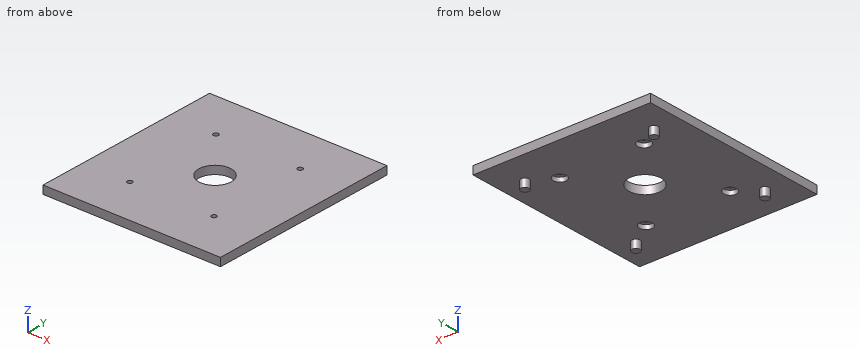
from build123d import *

# Parameters (mm, degrees)
F0_W           = 139.7
F0_H           = 152.4
F0_R           = 3.175
F0_R_2         = 1.984375
F0_R_3         = 12.7
F1_DEPTH       = 6.35
F2_R           = 3.175
F3_DEPTH       = 12.7
F5_D           = 3.9624
F5_CBORE_D     = 10.31875
F5_CBORE_DEPTH = 3.3734375


with BuildPart() as f1:
    # F0 (on Top) → F1 (new body)
    with BuildSketch(Plane.XY):
        Rectangle(F0_W, F0_H)
        with Locations((-50.8, -50.8)):
            Circle(F0_R, mode=Mode.SUBTRACT)
        with Locations((-25.4, -50.8)):
            Circle(F0_R, mode=Mode.SUBTRACT)
        with Locations((-33.1390625, -39.38984375)):
            Circle(F0_R_2, mode=Mode.SUBTRACT)
        with Locations((-50.8, -25.4)):
            Circle(F0_R, mode=Mode.SUBTRACT)
        with Locations((-25.4, -25.4)):
            Circle(F0_R, mode=Mode.SUBTRACT)
        with Locations((0, -50.8)):
            Circle(F0_R, mode=Mode.SUBTRACT)
        with Locations((25.4, -50.8)):
            Circle(F0_R, mode=Mode.SUBTRACT)
        with Locations((33.1390625, -39.38984375)):
            Circle(F0_R_2, mode=Mode.SUBTRACT)
        with Locations((50.8, -50.8)):
            Circle(F0_R, mode=Mode.SUBTRACT)
        with Locations((0, -25.4)):
            Circle(F0_R, mode=Mode.SUBTRACT)
        with Locations((25.4, -25.4)):
            Circle(F0_R, mode=Mode.SUBTRACT)
        with Locations((50.8, -25.4)):
            Circle(F0_R, mode=Mode.SUBTRACT)
        with Locations((-50.8, 0)):
            Circle(F0_R, mode=Mode.SUBTRACT)
        with Locations((-50.8, 25.4)):
            Circle(F0_R, mode=Mode.SUBTRACT)
        with Locations((-25.4, 0)):
            Circle(F0_R, mode=Mode.SUBTRACT)
        with Locations((-25.4, 25.4)):
            Circle(F0_R, mode=Mode.SUBTRACT)
        with Locations((-50.8, 50.8)):
            Circle(F0_R, mode=Mode.SUBTRACT)
        with Locations((-33.1390625, 39.38984375)):
            Circle(F0_R_2, mode=Mode.SUBTRACT)
        with Locations((-25.4, 50.8)):
            Circle(F0_R, mode=Mode.SUBTRACT)
        Circle(F0_R_3, mode=Mode.SUBTRACT)
        with Locations((25.4, 0)):
            Circle(F0_R, mode=Mode.SUBTRACT)
        with Locations((0, 25.4)):
            Circle(F0_R, mode=Mode.SUBTRACT)
        with Locations((25.4, 25.4)):
            Circle(F0_R, mode=Mode.SUBTRACT)
        with Locations((50.8, 0)):
            Circle(F0_R, mode=Mode.SUBTRACT)
        with Locations((50.8, 25.4)):
            Circle(F0_R, mode=Mode.SUBTRACT)
        with Locations((0, 50.8)):
            Circle(F0_R, mode=Mode.SUBTRACT)
        with Locations((33.1390625, 39.38984375)):
            Circle(F0_R_2, mode=Mode.SUBTRACT)
        with Locations((25.4, 50.8)):
            Circle(F0_R, mode=Mode.SUBTRACT)
        with Locations((50.8, 50.8)):
            Circle(F0_R, mode=Mode.SUBTRACT)
        with Locations((-25.4, 50.8)):
            Circle(F0_R)
        with Locations((0, 50.8)):
            Circle(F0_R)
        with Locations((25.4, 50.8)):
            Circle(F0_R)
        with Locations((50.8, 25.4)):
            Circle(F0_R)
        with Locations((50.8, 0)):
            Circle(F0_R)
        with Locations((50.8, -25.4)):
            Circle(F0_R)
        with Locations((25.4, -50.8)):
            Circle(F0_R)
        with Locations((0, -50.8)):
            Circle(F0_R)
        with Locations((-25.4, -50.8)):
            Circle(F0_R)
        with Locations((-50.8, -25.4)):
            Circle(F0_R)
        with Locations((-50.8, 0)):
            Circle(F0_R)
        with Locations((-50.8, 25.4)):
            Circle(F0_R)
        with Locations((-25.4, 25.4)):
            Circle(F0_R)
        with Locations((0, 25.4)):
            Circle(F0_R)
        with Locations((25.4, 25.4)):
            Circle(F0_R)
        with Locations((25.4, 0)):
            Circle(F0_R)
        with Locations((25.4, -25.4)):
            Circle(F0_R)
        with Locations((0, -25.4)):
            Circle(F0_R)
        with Locations((-25.4, 0)):
            Circle(F0_R)
        with Locations((-25.4, -25.4)):
            Circle(F0_R)
    extrude(amount=F1_DEPTH)

    # F2 (on face) → F3 (join)
    with BuildSketch(Plane.XY.offset(6.35)):
        with Locations((50.8, -50.8)):
            Circle(F2_R)
        with Locations((-50.8, -50.8)):
            Circle(F2_R)
        with Locations((-50.8, 50.8)):
            Circle(F2_R)
        with Locations((50.8, 50.8)):
            Circle(F2_R)
    extrude(amount=-F3_DEPTH)

    # F5 (through all)
    with Locations(Plane(origin=(0, 0, 0), x_dir=(1, 0, 0), z_dir=(0, 0, -1))):
        with Locations((-33.1390625, 39.38984375), (33.1390625, 39.38984375), (33.1390625, -39.38984375), (-33.1390625, -39.38984375)):
            CounterBoreHole(F5_D / 2, F5_CBORE_D / 2, F5_CBORE_DEPTH)


solid = f1.part
Could you check a few things on this model? Use its own coordinates, in mm. Round coordinates to 2 decimals unless told otherwise and drop trailing zeros. Write each loop counter-clockwise with the first axis right and the second up, starting at its lowest first coordinate (ties: lowest second). Pieces come first, ordered by that corner, then holes. Notation, with made-up numbers: (51, -28) -> (110, -28) arc R14 ccw to (110, -12) -> close; hole circle Ø11 at (-21, -13). An arc over 180 degrees is marked (long way). Use a Markdown table: item, result.
1. For pin 1 Ø5 at (x, y) = (-32.5, 41.5) entering from -Z; pin 2 Ø3 at (x, y) = (-33.14, -39.39) entering from -Z; pin 3 Ø16.5 at (x, y) = (-33.14, -39.39) entering from -Z, each with a flat end and sliding along its axis, tell me the tip position at first contact or that it passes through.
Answer key:
| item | result |
|---|---|
| pin 1 | stops at z = 3.37 |
| pin 2 | passes through |
| pin 3 | stops at z = 0 |
2. If we section it at A-A (y = 0): List the corners of the cut face in (x, z) for me, then the cut area to 3 significant figures.
Answer key:
| item | result |
|---|---|
| outline | (-69.85, 0) -> (-12.7, 0) -> (-12.7, 6.35) -> (-69.85, 6.35) -> close; (12.7, 0) -> (69.85, 0) -> (69.85, 6.35) -> (12.7, 6.35) -> close |
| area | 726 mm^2 |
3. Please list where these lines run through material, in increasing order: probe 1 along Y at (x, z) = (-34, 2.5); probe 2 along Y at (x, z) = (0, 3); probe 3 along Y at (x, z) = (36, 2).
Answer key:
| item | result |
|---|---|
| probe 1 | y = -76.2 to -44.48, -34.3 to 34.3, 44.48 to 76.2 |
| probe 2 | y = -76.2 to -12.7, 12.7 to 76.2 |
| probe 3 | y = -76.2 to -43.68, -35.1 to 35.1, 43.68 to 76.2 |
4. If we section it at B-B (z = -3.5): List the corners of the cut face in (x, y) for me (3 decimals), then the cut area to 3 significant figures.
Answer key:
| item | result |
|---|---|
| outline | circle Ø6.35 at (-50.8, -50.8); circle Ø6.35 at (-50.8, 50.8); circle Ø6.35 at (50.8, -50.8); circle Ø6.35 at (50.8, 50.8) |
| area | 127 mm^2 |
5. If we section it at C-C (x = 33): List the corners of the cut face in (y, z) for me.
Answer key:
| item | result |
|---|---|
| outline | (-76.2, 0) -> (-44.55, 0) -> (-44.55, 3.37) -> (-41.37, 3.37) -> (-41.37, 6.35) -> (-76.2, 6.35) -> close; (-37.41, 3.37) -> (-34.23, 3.37) -> (-34.23, 0) -> (34.23, 0) -> (34.23, 3.37) -> (37.41, 3.37) -> (37.41, 6.35) -> (-37.41, 6.35) -> close; (41.37, 3.37) -> (44.55, 3.37) -> (44.55, 0) -> (76.2, 0) -> (76.2, 6.35) -> (41.37, 6.35) -> close |
6. If we section it at D-D (y = 50.8): List the corners of the cut face in (x, z) for me (3 decimals).
Answer key:
| item | result |
|---|---|
| outline | (-69.85, 0) -> (-53.975, 0) -> (-53.975, -6.35) -> (-47.625, -6.35) -> (-47.625, 0) -> (47.625, 0) -> (47.625, -6.35) -> (53.975, -6.35) -> (53.975, 0) -> (69.85, 0) -> (69.85, 6.35) -> (-69.85, 6.35) -> close |
